from build123d import *

# Parameters (mm, degrees)
SKETCH1_W                    = 120
SKETCH1_H                    = 65
BOSS_EXTRUDE1_DEPTH          = 5
SKETCH2_W                    = 115
SKETCH2_H                    = 60
BOSS_EXTRUDE2_DEPTH          = 2.5
F_5_0_5_DIAMETER_HOLE1_D     = 5
F_5_0_5_DIAMETER_HOLE1_DEPTH = 7.5
SKETCH5_W                    = 111
SKETCH5_H                    = 56
CUT_EXTRUDE3_DEPTH           = 6.12


with BuildPart() as part:
    # Sketch1 → Boss-Extrude1 (new body)
    with BuildSketch(Plane.XY.offset(2.5)):
        with Locations((60, 32.5)):
            Rectangle(SKETCH1_W, SKETCH1_H)
    extrude(amount=-BOSS_EXTRUDE1_DEPTH)

    # Sketch2 → Boss-Extrude2 (add)
    with BuildSketch(Plane.XY.offset(2.5)):
        with Locations((60, 32.5)):
            Rectangle(SKETCH2_W, SKETCH2_H)
    extrude(amount=BOSS_EXTRUDE2_DEPTH)

    # Ø5.0 (5) Diameter Hole1
    with Locations(Plane(origin=(0, 0, -2.5), x_dir=(-1, 0, 0), z_dir=(0, 0, -1))):
        with Locations((-8.5, 38)):
            Hole(F_5_0_5_DIAMETER_HOLE1_D / 2, depth=F_5_0_5_DIAMETER_HOLE1_DEPTH)

    # Sketch5 → Cut-Extrude3 (cut)
    with BuildSketch(Plane.XY.offset(5)):
        with Locations((60, 32.5)):
            Rectangle(SKETCH5_W, SKETCH5_H)
    extrude(amount=-CUT_EXTRUDE3_DEPTH, mode=Mode.SUBTRACT)


solid = part.part
Geometry check sheet. Reference: the model listing, model coordinates, mm. A direction names the side the tool comes from. Round coordinates to 2 decimals unless told otherwise and drop trailing zeros. Order: outer loops, then holes, each group sorted by start corner. A loop starts at its lowest first (then second) coordinate and runs counter-clockwise, first axis right, second up. Notation, with made-up numbers: M -10,-19.5 L 41,-19.5 A11 ccw 41,-15.5 Z; hole C -18,45 d11. An arc over 180 degrees is marked long. Write each question's results on one line, items separated by ' | '. Start each with the question number.
1. Material ranges on L1, parallel to X at y = 39, z = 3.25; L2, parallel to Y at x = 8.5, z = -1.8; L3, parallel to Y at x = 61, z = 0.75, recorded low to high. Write a range as from..to.
2. Draft check along Y on faces 1 (the face through (59, 33, -1.12)), 2 (the face through (59, 2.5, 4)), 3 (the face through (0, 32, 0)). Enter one of: pulls with the +Y half, pulls with the -Y half, needs draft (parallel to the pull), parting line crosses it, or undercut.
3. Cross-section at C-C on x = 31.5. Record the boundary of the cut face in (y, z).
4. Set-up check for faces 4 (the face through (2.5, 32, 4)), 5 (the face through (59, 62.5, 4)), 6 (the face through (117.5, 32, 4)), 7 (the face through (4.5, 32, 2)): record each of +Z, -Z, +X, -X, +Y, -Y from which the full face is reachable in a straight line by a thin tool's end or side.
5. Cross-section at B-B on x = 8.5. Record the boundary of the cut face in (y, z), plus the area to 3 significant figures.
6. Cross-section at A-A on y = 38. Record the boundary of the cut face in (x, z).
7. Cross-section at D-D on y = 48. Record the boundary of the cut face in (x, z).
8. Go/stop test with flat-tipped pins: P1, Ø1.8, axis at x = 86, z = 3.5, coming from the +Y side; P2, Ø1.5, axis at x = 18, y = 48.5, coming from the +Z side; P3, Ø0.8, axis at x = 72.5, z = 3, coming from the -Y side. Record where each tip stops, or that it passes through.
Resolved:
1) L1: 2.5..4.5, 115.5..117.5 | L2: 0..35.5, 40.5..65 | L3: 0..4.5, 60.5..65
2) face 1: undercut | face 2: pulls with the -Y half | face 3: needs draft
3) outline: M 0,-2.5 L 65,-2.5 L 65,2.5 L 62.5,2.5 L 62.5,5 L 60.5,5 L 60.5,-1.12 L 4.5,-1.12 L 4.5,5 L 2.5,5 L 2.5,2.5 L 0,2.5 Z
4) face 4: +Z, -X, +Y, -Y | face 5: +Z, +X, -X, +Y | face 6: +Z, +X, +Y, -Y | face 7: +Z
5) outline: M 0,-2.5 L 35.5,-2.5 L 35.5,-1.12 L 4.5,-1.12 L 4.5,5 L 2.5,5 L 2.5,2.5 L 0,2.5 Z; M 40.5,-2.5 L 65,-2.5 L 65,2.5 L 62.5,2.5 L 62.5,5 L 60.5,5 L 60.5,-1.12 L 40.5,-1.12 Z | area: 125 mm2
6) outline: M 0,-2.5 L 6,-2.5 L 6,-1.12 L 4.5,-1.12 L 4.5,5 L 2.5,5 L 2.5,2.5 L 0,2.5 Z; M 11,-2.5 L 120,-2.5 L 120,2.5 L 117.5,2.5 L 117.5,5 L 115.5,5 L 115.5,-1.12 L 11,-1.12 Z
7) outline: M 0,-2.5 L 120,-2.5 L 120,2.5 L 117.5,2.5 L 117.5,5 L 115.5,5 L 115.5,-1.12 L 4.5,-1.12 L 4.5,5 L 2.5,5 L 2.5,2.5 L 0,2.5 Z
8) P1: y = 62.5 | P2: z = -1.12 | P3: y = 2.5
